Could you check a few things on this model? Use its own coordinates, in mm. A direction names the side the tool comes from. Round coordinates to 2 decimals unless told otherwise and drop trailing zeros. Write each loop counter-clockwise with the first axis right and the second up, starting at its lowest first coordinate (ties: lowest second). Pieces come first, ordered by that corner, then holes. Notation, with made-up numbers: (-26.5, 39.25) -> (11.5, 39.25) arc R15 ccw to (11.5, 64.25) -> close; hole circle Ø3 at (-28.5, 2.5). An arc over 180 degrees is marked (long way). Answer in a Markdown table with one row per item.
from build123d import *

# Parameters (mm, degrees)
BOX004_W               = 1.5
BOX004_H               = 14.7
BOX004_DEPTH           = 3
CHAMFER001_SIZE        = 1.49
BOX005_W               = 1.5
BOX005_H               = 14.7
BOX005_DEPTH           = 3
CHAMFER002_SIZE        = 1.49
BOX006_W               = 1.5
BOX006_H               = 14.7
BOX006_DEPTH           = 3
CHAMFER003_SIZE        = 1.49
EXTRUDE006_DEPTH       = 3
EXTRUDE005_DEPTH       = 3
BOX001_W               = 100
BOX001_H               = 100
BOX001_DEPTH           = 100
BOX001_PLACEMENT_ANGLE = 30
BOX_W                  = 100
BOX_H                  = 100
BOX_DEPTH              = 100
BOX_PLACEMENT_ANGLE    = 30
EXTRUDE_DEPTH          = 2
EXTRUDE001_DEPTH       = 2
EXTRUDE002_DEPTH       = 10
EXTRUDE003_DEPTH       = 52
EXTRUDE004_DEPTH       = 56
BOX002_W               = 100
BOX002_H               = 2
BOX002_DEPTH           = 100
BOX002_PLACEMENT_ANGLE = 30
BOX003_W               = 1.5
BOX003_H               = 14.7
BOX003_DEPTH           = 3
CHAMFER_SIZE           = 1.49


with BuildPart() as chamfer001:
    # Box004 → Box004 (new body)
    with BuildSketch(Plane(origin=(-45.25, -29, 8), x_dir=(1, 0, 0), z_dir=(0, 0, 1))):
        with Locations((0.75, 7.35)):
            Rectangle(BOX004_W, BOX004_H)
    extrude(amount=BOX004_DEPTH)

    # Chamfer001
    chamfer001_edges = [chamfer001.edges().sort_by_distance(p)[0] for p in [
        (-43.75, -29, 9.5),
        (-43.75, -21.65, 11),
        (-43.75, -14.3, 9.5),
        (-43.75, -21.65, 8),
    ]]
    chamfer(chamfer001_edges, length=CHAMFER001_SIZE)


with BuildPart() as chamfer002:
    # Box005 → Box005 (new body)
    with BuildSketch(Plane(origin=(43.75, 10, 7), x_dir=(1, 0, 0), z_dir=(0, 0, 1))):
        with Locations((0.75, 7.35)):
            Rectangle(BOX005_W, BOX005_H)
    extrude(amount=BOX005_DEPTH)

    # Chamfer002
    chamfer002_edges = [chamfer002.edges().sort_by_distance(p)[0] for p in [
        (43.75, 10, 8.5),
        (43.75, 17.35, 10),
        (43.75, 24.7, 8.5),
        (43.75, 17.35, 7),
    ]]
    chamfer(chamfer002_edges, length=CHAMFER002_SIZE)


with BuildPart() as chamfer003:
    # Box006 → Box006 (new body)
    with BuildSketch(Plane(origin=(-45.25, 10, 8), x_dir=(1, 0, 0), z_dir=(0, 0, 1))):
        with Locations((0.75, 7.35)):
            Rectangle(BOX006_W, BOX006_H)
    extrude(amount=BOX006_DEPTH)

    # Chamfer003
    chamfer003_edges = [chamfer003.edges().sort_by_distance(p)[0] for p in [
        (-43.75, 10, 9.5),
        (-43.75, 17.35, 11),
        (-43.75, 24.7, 9.5),
        (-43.75, 17.35, 8),
    ]]
    chamfer(chamfer003_edges, length=CHAMFER003_SIZE)


with BuildPart() as extrude006:
    # Sketch007 (on Face25 of Cut001) → Extrude006 (new body)
    with BuildSketch(Plane(origin=(-47.25, 0, 0), x_dir=(0, -1, 0), z_dir=(-1, 0, 0))):
        with BuildLine():
            ThreePointArc((0.75, 10.5), (-2.75, 7), (0.75, 3.5))
            Line((0.75, 3.5), (7.75, 3.5))
            ThreePointArc((7.75, 3.5), (11.25, 7), (7.75, 10.5))
            Line((7.75, 10.5), (0.75, 10.5))
        make_face()
    extrude(amount=-EXTRUDE006_DEPTH)


with BuildPart() as extrude005:
    # Sketch006 (on Face43 of Cut001) → Extrude005 (new body)
    with BuildSketch(Plane.XZ.offset(33)):
        with BuildLine():
            ThreePointArc((2, 5.5), (3.5, 7), (2, 8.5))
            Line((2, 8.5), (-11, 8.5))
            ThreePointArc((-11, 8.5), (-12.5, 7), (-11, 5.5))
            Line((-11, 5.5), (2, 5.5))
        make_face()
    extrude(amount=-EXTRUDE005_DEPTH)


with BuildPart() as cube001:
    # Box001 → Box001 (new body)
    with BuildSketch(Plane.XY):
        with Locations((50, 50)):
            Rectangle(BOX001_W, BOX001_H)
    extrude(amount=BOX001_DEPTH)


with BuildPart() as cube001_1:
    # Box001 placement: moved
    add(cube001.part.moved(Location((-50, -49.539727, 19.087357))).rotate(Axis((-50, -49.539727, 19.087357), (1, 0, 0)), BOX001_PLACEMENT_ANGLE))


with BuildPart() as cube:
    # Box → Box (new body)
    with BuildSketch(Plane.XY):
        with Locations((50, 50)):
            Rectangle(BOX_W, BOX_H)
    extrude(amount=BOX_DEPTH)


with BuildPart() as cube_1:
    # Box placement: moved
    add(cube.part.moved(Location((-50, 39.30718, -0.4))).rotate(Axis((-50, 39.30718, -0.4), (1, 0, 0)), BOX_PLACEMENT_ANGLE))


with BuildPart() as extrude_body:
    # Sketch001 → Extrude (new body)
    with BuildSketch(Plane.XY):
        with BuildLine():
            ThreePointArc((-39.75, 33), (-45.053301, 30.803301), (-47.25, 25.5))
            Line((-47.25, -25.5), (-47.25, 25.5))
            ThreePointArc((-47.25, -25.5), (-45.053301, -30.803301), (-39.75, -33))
            Line((39.75, -33), (-39.75, -33))
            ThreePointArc((39.75, -33), (45.053301, -30.803301), (47.25, -25.5))
            Line((47.25, 25.5), (47.25, -25.5))
            ThreePointArc((47.25, 25.5), (45.053301, 30.803301), (39.75, 33))
            Line((-39.75, 33), (39.75, 33))
        make_face()
        with BuildLine():
            ThreePointArc((-39.75, 23.4), (-43.639087, 21.789087), (-45.25, 17.9))
            Line((-45.25, -25.5), (-45.25, 17.9))
            ThreePointArc((-45.25, -25.5), (-43.639087, -29.389087), (-39.75, -31))
            Line((39.75, -31), (-39.75, -31))
            ThreePointArc((39.75, -31), (43.639087, -29.389087), (45.25, -25.5))
            Line((45.25, 17.9), (45.25, -25.5))
            ThreePointArc((45.25, 17.9), (43.639087, 21.789087), (39.75, 23.4))
            Line((-39.75, 23.4), (39.75, 23.4))
        make_face(mode=Mode.SUBTRACT)
    extrude(amount=EXTRUDE_DEPTH)


with BuildPart() as extrude_2mm:
    # Sketch002 → Extrude001 (new body)
    with BuildSketch(Plane.XY.offset(2)):
        with BuildLine():
            ThreePointArc((-39.75, 33), (-45.053301, 30.803301), (-47.25, 25.5))
            Line((-47.25, -25.5), (-47.25, 25.5))
            ThreePointArc((-47.25, -25.5), (-45.053301, -30.803301), (-39.75, -33))
            Line((39.75, -33), (-39.75, -33))
            ThreePointArc((39.75, -33), (45.053301, -30.803301), (47.25, -25.5))
            Line((47.25, 25.5), (47.25, -25.5))
            ThreePointArc((47.25, 25.5), (45.053301, 30.803301), (39.75, 33))
            Line((-39.75, 33), (39.75, 33))
        make_face()
        with BuildLine():
            ThreePointArc((-39.75, 23.4), (-43.639087, 21.789087), (-45.25, 17.9))
            Line((-45.25, -25.5), (-45.25, 17.9))
            ThreePointArc((-45.25, -25.5), (-43.639087, -29.389087), (-39.75, -31))
            Line((39.75, -31), (-39.75, -31))
            ThreePointArc((39.75, -31), (43.639087, -29.389087), (45.25, -25.5))
            Line((45.25, 17.9), (45.25, -25.5))
            ThreePointArc((45.25, 17.9), (43.639087, 21.789087), (39.75, 23.4))
            Line((-39.75, 23.4), (39.75, 23.4))
        make_face(mode=Mode.SUBTRACT)
        with BuildLine():
            ThreePointArc((-39.75, 31), (-43.639087, 29.389087), (-45.25, 25.5))
            Line((-45.25, 25.5), (-45.25, 25.4))
            Line((-45.25, 25.4), (45.25, 25.4))
            Line((45.25, 25.5), (45.25, 25.4))
            ThreePointArc((45.25, 25.5), (43.639086, 29.389089), (39.749996, 31))
            Line((-39.75, 31), (39.749996, 31))
        make_face(mode=Mode.SUBTRACT)
    extrude(amount=EXTRUDE001_DEPTH)


with BuildPart() as extrude_4mm:
    # Sketch003 → Extrude002 (new body)
    with BuildSketch(Plane.XY.offset(4)):
        with BuildLine():
            ThreePointArc((-39.75, 33), (-45.053301, 30.803301), (-47.25, 25.5))
            Line((-47.25, -25.5), (-47.25, 25.5))
            ThreePointArc((-47.25, -25.5), (-45.053301, -30.803301), (-39.75, -33))
            Line((39.75, -33), (-39.75, -33))
            ThreePointArc((39.75, -33), (45.053301, -30.803301), (47.25, -25.5))
            Line((47.25, 25.5), (47.25, -25.5))
            ThreePointArc((47.25, 25.5), (45.053301, 30.803301), (39.75, 33))
            Line((-39.75, 33), (39.75, 33))
        make_face()
        with BuildLine():
            ThreePointArc((-39.75, 31), (-43.639087, 29.389087), (-45.25, 25.5))
            Line((-45.25, -25.5), (-45.25, 25.5))
            ThreePointArc((-45.25, -25.5), (-43.639087, -29.389087), (-39.75, -31))
            Line((39.75, -31), (-39.75, -31))
            ThreePointArc((39.75, -31), (43.639087, -29.389087), (45.25, -25.5))
            Line((45.25, 25.5), (45.25, -25.5))
            ThreePointArc((45.25, 25.5), (43.639087, 29.389087), (39.75, 31))
            Line((-39.75, 31), (39.75, 31))
        make_face(mode=Mode.SUBTRACT)
    extrude(amount=EXTRUDE002_DEPTH)


with BuildPart() as extrude_6mm:
    # Sketch003 → Extrude003 (new body)
    with BuildSketch(Plane.XY.offset(4)):
        with BuildLine():
            ThreePointArc((-39.75, 33), (-45.053301, 30.803301), (-47.25, 25.5))
            Line((-47.25, -25.5), (-47.25, 25.5))
            ThreePointArc((-47.25, -25.5), (-45.053301, -30.803301), (-39.75, -33))
            Line((39.75, -33), (-39.75, -33))
            ThreePointArc((39.75, -33), (45.053301, -30.803301), (47.25, -25.5))
            Line((47.25, 25.5), (47.25, -25.5))
            ThreePointArc((47.25, 25.5), (45.053301, 30.803301), (39.75, 33))
            Line((-39.75, 33), (39.75, 33))
        make_face()
        with BuildLine():
            ThreePointArc((-39.75, 31), (-43.639087, 29.389087), (-45.25, 25.5))
            Line((-45.25, -25.5), (-45.25, 25.5))
            ThreePointArc((-45.25, -25.5), (-43.639087, -29.389087), (-39.75, -31))
            Line((39.75, -31), (-39.75, -31))
            ThreePointArc((39.75, -31), (43.639087, -29.389087), (45.25, -25.5))
            Line((45.25, 25.5), (45.25, -25.5))
            ThreePointArc((45.25, 25.5), (43.639087, 29.389087), (39.75, 31))
            Line((-39.75, 31), (39.75, 31))
        make_face(mode=Mode.SUBTRACT)
    extrude(amount=EXTRUDE003_DEPTH)


with BuildPart() as extrude004:
    # Sketch004 → Extrude004 (new body)
    with BuildSketch(Plane.XY):
        with BuildLine():
            ThreePointArc((-39.75, 33), (-45.053301, 30.803301), (-47.25, 25.5))
            Line((-47.25, -25.5), (-47.25, 25.5))
            ThreePointArc((-47.25, -25.5), (-45.053301, -30.803301), (-39.75, -33))
            Line((39.75, -33), (-39.75, -33))
            ThreePointArc((39.75, -33), (45.053301, -30.803301), (47.25, -25.5))
            Line((47.25, 25.5), (47.25, -25.5))
            ThreePointArc((47.25, 25.5), (45.053301, 30.803301), (39.75, 33))
            Line((-39.75, 33), (39.75, 33))
        make_face()
    extrude(amount=EXTRUDE004_DEPTH)


with BuildPart() as cut003:
    # Box002 → Box002 (new body)
    with BuildSketch(Plane.XY):
        with Locations((50, 1)):
            Rectangle(BOX002_W, BOX002_H)
    extrude(amount=BOX002_DEPTH)


with BuildPart() as cut003_1:
    # Box002 placement: moved
    add(cut003.part.moved(Location((-50, 37.575129, -1.4))).rotate(Axis((-50, 37.575129, -1.4), (1, 0, 0)), BOX002_PLACEMENT_ANGLE))

    # Common: intersect Extrude004
    add(extrude004.part, mode=Mode.INTERSECT)

    # Fusion: union Extrude body, Extrude_2mm, Extrude_4mm, Extrude_6mm
    add(extrude_body.part)
    add(extrude_2mm.part)
    add(extrude_4mm.part)
    add(extrude_6mm.part)

    # Cut: cut Cube
    add(cube_1.part, mode=Mode.SUBTRACT)

    # Cut001: cut Cube001
    add(cube001_1.part, mode=Mode.SUBTRACT)

    # Cut002: cut Extrude005
    add(extrude005.part, mode=Mode.SUBTRACT)

    # Cut003: cut Extrude006
    add(extrude006.part, mode=Mode.SUBTRACT)


with BuildPart() as main:
    # Box003 → Box003 (new body)
    with BuildSketch(Plane(origin=(43.75, -29, 7), x_dir=(1, 0, 0), z_dir=(0, 0, 1))):
        with Locations((0.75, 7.35)):
            Rectangle(BOX003_W, BOX003_H)
    extrude(amount=BOX003_DEPTH)

    # Chamfer
    chamfer_edges = [main.edges().sort_by_distance(p)[0] for p in [
        (43.75, -29, 8.5),
        (43.75, -21.65, 10),
        (43.75, -14.3, 8.5),
        (43.75, -21.65, 7),
    ]]
    chamfer(chamfer_edges, length=CHAMFER_SIZE)

    # Connect: union Chamfer001, Chamfer002, Chamfer003, Cut003
    add(chamfer001.part)
    add(chamfer002.part)
    add(chamfer003.part)
    add(cut003_1.part)


solid = main.part
1) Thinking about a two-plate mould opening in X: for faces 1 (the face through (-45.25, 0, 20)), 2 (the face through (1, -33, 14)), 3 (the face through (44.995, -30.861, 16.253)), which applies, +X half, -X half, draft (parallel to the pull), parting line (faces both ways), or undercut?
Findings:
| item | result |
|---|---|
| face 1 | undercut |
| face 2 | draft |
| face 3 | +X half |
2) Please list where these lines run through material, in increasing order: line 1 (X direction, y = -13.5, z = 37.5); line 2 (Y direction, x = 12.5, z = 7.5); line 3 (Y direction, x = 40, z = 21).
Findings:
| item | result |
|---|---|
| line 1 | x = -47.25 to -45.25, 45.25 to 47.25 |
| line 2 | y = -33 to -31, 31 to 33 |
| line 3 | y = -33 to -30.99, 24.64 to 26.95 |
3) For pin 1 (1.6 mm diameter, centred on x = -46.5, y = -5, fed in from +Z); pin 2 (1.6 mm diameter, centred on x = -2.5, y = -32, fed in from +Z); pin 3 (6 mm diameter, centred on x = -20, z = 41, fed in from -Y), each with a flat end and sliding along its axis, tell me the tip position at first contact or that it passes through.
Findings:
| item | result |
|---|---|
| pin 1 | stops at z = 45.26 |
| pin 2 | stops at z = 29.68 |
| pin 3 | stops at y = 11.36 |
4) For faces 4 (the face through (-43.6, 21.83, 1.97)), 5 (the face through (-1, 31, 6)), 6 (the face through (-46, -4, 3.5)), which set-ups out of +Z, -Z, +X, -X, +Y, -Y let a thin tool reach every point of the face, with its end or its side?
Findings:
| item | result |
|---|---|
| face 4 | -Z |
| face 5 | none |
| face 6 | -X |
5) Imagine slicing it at C-C, the plane y = -10. Please give me the cut outline in (x, z), plus the area to 3 significant figures.
Findings:
| item | result |
|---|---|
| outline | (-47.25, 0) -> (-45.25, 0) -> (-45.25, 4.32) -> (-47.25, 4.32) -> close; (-47.25, 9.68) -> (-45.25, 9.68) -> (-45.25, 41.92) -> (-47.25, 41.92) -> close; (45.25, 0) -> (47.25, 0) -> (47.25, 41.92) -> (45.25, 41.92) -> close |
| area | 157 mm^2 |
6) Imagine slicing it at D-D, the plane z = 44.5. Please give me the cut outline in (x, y), plus the area to 3 significant figures.
Findings:
| item | result |
|---|---|
| outline | (-47.25, -5.52) -> (-45.25, -5.52) -> (-45.25, 11.07) -> (45.25, 11.07) -> (45.25, -5.52) -> (47.25, -5.52) -> (47.25, 13.38) -> (-47.25, 13.38) -> close |
| area | 285 mm^2 |
7) Imagine slicing it at B-B, the plane z = 22. Please give me the cut outline in (x, y), plus the area to 3 significant figures.
Findings:
| item | result |
|---|---|
| outline | (-47.25, -25.5) arc R7.5 ccw to (-39.75, -33) -> (39.75, -33) arc R7.5 ccw to (47.25, -25.5) -> (47.25, 25.5) arc R7.5 ccw to (47.2, 26.37) -> (-47.2, 26.37) arc R7.5 ccw to (-47.25, 25.5) -> close; hole (-45.25, -25.5) arc R5.5 ccw to (-39.75, -31) -> (39.75, -31) arc R5.5 ccw to (45.25, -25.5) -> (45.25, 24.07) -> (-45.25, 24.07) -> close |
| area | 616 mm^2 |
8) Imagine slicing it at A-A, the plane x = 38. Please give me the cut outline in (y, z).
Findings:
| item | result |
|---|---|
| outline | (-33, 0) -> (-31, 0) -> (-31, 29.79) -> (-33, 28.64) -> close; (6.93, 51.69) -> (31, 9.99) -> (31, 2) -> (25.4, 2) -> (25.4, 4) -> (23.4, 4) -> (23.4, 0) -> (33, 0) -> (33, 10.52) -> (8.66, 52.69) -> close |
